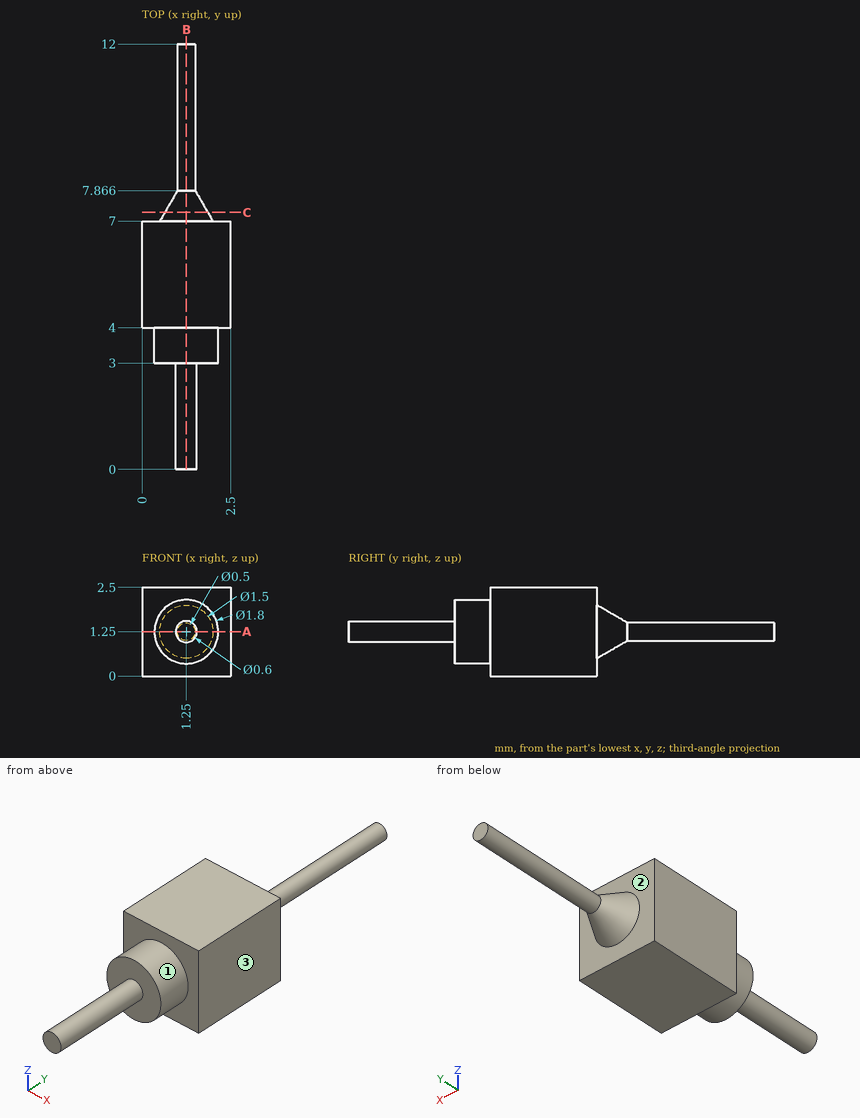
Can you work these out from the drawing? Everything is in mm from the part's minimum corner. A direction names the side the tool comes from. Give positions to 0.01 mm unless a question says otherwise; leave off trailing zeros. Write each loop counter-clockwise with the first axis right and the second up, starting at its lowest first coordinate (ties: lowest second). Pieces come first, ordered by that corner, then holes. Notation, with made-up numbers: (9.25, -11) -> (58.25, -11) arc R32 ccw to (58.25, 23) -> close; hole circle Ø10 at (82, 61). An arc over 180 degrees is marked (long way). Write each question's results on one line, items separated by ' | '.
Item 1: Suppose I cut it at A-A on z = 1.25. Write out the boundary of the cut face in (x, y).
Output:
outline: (0, 4) -> (0.35, 4) -> (0.35, 3) -> (0.95, 3) -> (0.95, 0) -> (1.55, 0) -> (1.55, 3) -> (2.15, 3) -> (2.15, 4) -> (2.5, 4) -> (2.5, 7) -> (2, 7) -> (1.5, 7.87) -> (1.5, 12) -> (1, 12) -> (1, 7.87) -> (0.5, 7) -> (0, 7) -> close
Item 2: Suppose I cut it at B-B on x = 1.25. Write out the boundary of the cut face in (y, z).
Output:
outline: (0, 0.95) -> (3, 0.95) -> (3, 0.35) -> (4, 0.35) -> (4, 0) -> (7, 0) -> (7, 0.5) -> (7.87, 1) -> (12, 1) -> (12, 1.5) -> (7.87, 1.5) -> (7, 2) -> (7, 2.5) -> (4, 2.5) -> (4, 2.15) -> (3, 2.15) -> (3, 1.55) -> (0, 1.55) -> close
Item 3: For pin 1 Ø1 at (y, z) = (1, 1) entering from +X; pin 2 Ø1.5 at (y, z) = (9, 1.5) entering from -X, each with a flat end and sliding along its axis, tell me the tip position at first contact or that it passes through.
Output:
pin 1: stops at x = 1.55 | pin 2: stops at x = 1
Item 4: If I drill on L1, parallel to Y at x = 0.65, z = 0.65; L2, parallel to Y at x = 0.4, z = 1.95; L3, parallel to Z at x = 1.25, y = 10.5, over which ranges is the centre line in solid material (lowest first)?
Output:
L1: y = 3 to 7 | L2: y = 4 to 7 | L3: z = 1 to 1.5
Item 5: On a 3-axis mill with a long thin cutter (end or side, diameter ignored), from which of +Z, -Z, +X, -X, +Y, -Y can I reach the whole of each face in a straight line? I mean the marked faces 1, 2 and 3. Say none if no direction works.
Output:
face 1: -Y | face 2: +Y | face 3: +Z, -Z, +X, +Y, -Y
Item 6: Suppose I cut it at C-C on y = 7.25. Write out the boundary of the cut face in (x, z).
Output:
outline: circle Ø1.21 at (1.25, 1.25)
